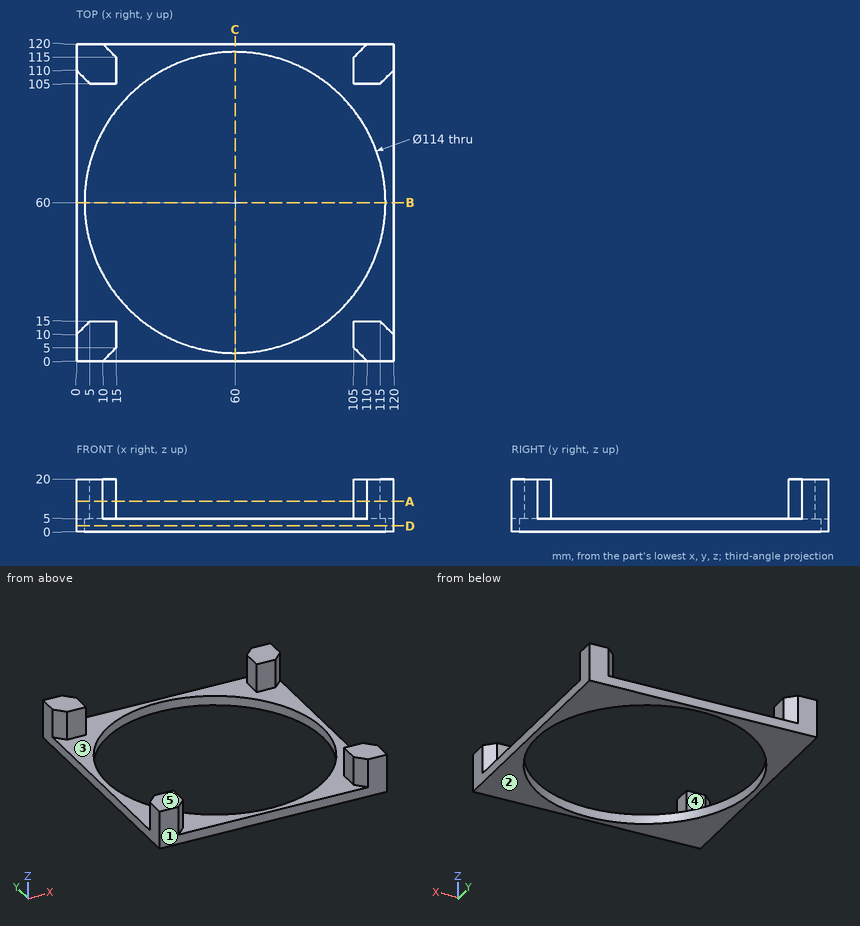
For this review, use the dimensioned drawing (mm, ordinates from the lowest corner) and the shaded views. A direction names the side the tool comes from. Round coordinates to 2 decimals unless told otherwise and drop trailing zeros. Write each loop counter-clockwise with the first axis right and the second up, starting at its lowest first coordinate (ties: lowest second). Pieces come first, ordered by that corner, then holes. Notation, with made-up numbers: (86.25, 43) - (116.25, 43) arc R24 cw to (116.25, 58) - close; hole circle Ø2 at (45.5, -11). An arc over 180 degrees is marked (long way). Use a Markdown table: item, result.
Q1. Clearance check with flat-ended pins moving along their axes: pin 1 (1 mm diameter, centred on x = 106.5, z = 17.5, fed in from +Y); pin 2 (11 mm diameter, centred on y = 112.5, z = 12, fed in from -X); pin 3 (3 mm diameter, centred on x = 107.5, z = 10.5, fed in from -Y); pin 4 (1 mm diameter, centred on x = 12, z = 16, fed in from +Y). State where each tip first meets the part, or that it passes through.
Derived:
| item | result |
|---|---|
| pin 1 | stops at y = 117 |
| pin 2 | stops at x = 0 |
| pin 3 | stops at y = 1 |
| pin 4 | stops at y = 118.5 |
Q2. We need section B-B (y = 60). Give the boundary of the cut face in (x, z), plus the area to 3 significant figures.
Derived:
| item | result |
|---|---|
| outline | (0, 0) - (3, 0) - (3, 5) - (0, 5) - close; (117, 0) - (120, 0) - (120, 5) - (117, 5) - close |
| area | 30.0 mm2 |
Q3. Machinability: for the marked faces 4 and 5, which of the approach directions +Z, -Z, +X, -X, +Y, -Y give a long, thin tool a straight path to every point of the face, cutting with its end or side? Answer none if there is none.
Derived:
| item | result |
|---|---|
| face 4 | +Z, +X, -X |
| face 5 | +Z, +X, -X, +Y, -Y |
Q4. We need section D-D (z = 2.25). Give the boundary of the cut face in (x, y), plus the area to 3 significant figures.
Derived:
| item | result |
|---|---|
| outline | (0, 0) - (120, 0) - (120, 120) - (0, 120) - close; hole circle Ø114 at (60, 60) |
| area | 4,190 mm2 |
Q5. The part is to be moulded in two halves that separate along Y. For the marked faces 1, 2 and 3, say which applies: pulls with the +Y half, pulls with the -Y half, needs draft (parallel to the pull), parting line crosses it, or undercut.
Derived:
| item | result |
|---|---|
| face 1 | pulls with the -Y half |
| face 2 | needs draft |
| face 3 | undercut |
Q6. We need section A-A (z = 11.5). Give the boundary of the cut face in (x, y), plus the area to 3 significant figures.
Derived:
| item | result |
|---|---|
| outline | (0, 0) - (10, 0) - (15, 5) - (15, 15) - (5, 15) - (0, 10) - close; (0, 110) - (5, 105) - (15, 105) - (15, 115) - (10, 120) - (0, 120) - close; (105, 5) - (110, 0) - (120, 0) - (120, 10) - (115, 15) - (105, 15) - close; (105, 105) - (115, 105) - (120, 110) - (120, 120) - (110, 120) - (105, 115) - close |
| area | 800 mm2 |
Q7. Wall thickness on line 1 along Y through (x, z) = (60, 3.4); line 2 along X through (y, z) = (13, 16.5); line 3 along X through (y, z) = (110.5, 17.5): over which ranges is each line inside the solid? List them lowest first.
Derived:
| item | result |
|---|---|
| line 1 | y = 0 to 3, 117 to 120 |
| line 2 | x = 3 to 15, 105 to 117 |
| line 3 | x = 0 to 15, 105 to 120 |
